Part model, mm, in its own coordinate system. Give positions to 0.01 mm unless a question says otherwise; leave off trailing zeros. Answer as a JSON object with one key per item and string values.
from build123d import *

# Parameters (mm, degrees)
SKETCH_1_R      = 2.5
SKETCH_1_W      = 3.3
SKETCH_1_H      = 3.3
EXTRUDE_1_DEPTH = 1445


with BuildPart() as part:
    # Эскиз1 → Бобышка-Вытянуть1 (new body)
    with BuildSketch(Plane.XY):
        Polygon((-10, 10), (-4.75, 10), (-3.1, 8), (-4.95, 8), (-4.95, 5.85), (-2.6, 3.5), (2.6, 3.5), (4.95, 5.85), (4.95, 8), (3.1, 8), (4.75, 10), (10, 10), (10, 4.75), (8, 3.1), (8, 4.95), (5.85, 4.95), (3.5, 2.6), (3.5, -2.6), (5.85, -4.95), (8, -4.95), (8, -3.1), (10, -4.75), (10, -10), (4.75, -10), (3.1, -8), (4.95, -8), (4.95, -5.85), (2.6, -3.5), (-2.6, -3.5), (-4.95, -5.85), (-4.95, -8), (-3.1, -8), (-4.75, -10), (-10, -10), (-10, -4.75), (-8, -3.1), (-8, -4.95), (-5.85, -4.95), (-3.5, -2.6), (-3.5, 2.6), (-5.85, 4.95), (-8, 4.95), (-8, 3.1), (-10, 4.75), align=None)
        Circle(SKETCH_1_R, mode=Mode.SUBTRACT)
        with Locations((-7.5, 7.5)):
            Rectangle(SKETCH_1_W, SKETCH_1_H, mode=Mode.SUBTRACT)
        with Locations((7.5, 7.5)):
            Rectangle(SKETCH_1_W, SKETCH_1_H, mode=Mode.SUBTRACT)
        with Locations((7.5, -7.5)):
            Rectangle(SKETCH_1_W, SKETCH_1_H, mode=Mode.SUBTRACT)
        with Locations((-7.5, -7.5)):
            Rectangle(SKETCH_1_W, SKETCH_1_H, mode=Mode.SUBTRACT)
    extrude(amount=-EXTRUDE_1_DEPTH)


solid = part.part
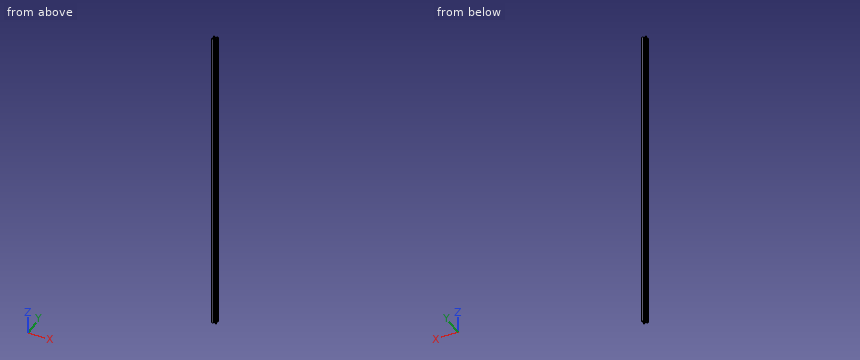
1. Cut at A-A on z = -617.5. State how many separate pieces and enclosed holes the cut face has, plus the area to 3 significant figures.
Worked answers:
{"separate pieces": "1", "enclosed holes": "5", "area": "118 mm^2"}
2. Pin check, flat tips, straight feed: P1, Ø3, axis at x = -2.5, z = -476, coming from the -Y side; P2, Ø1.6, axis at y = 1, z = -789.5, coming from the +X side; P3, Ø4, axis at y = 0.5, z = -952, coming from the -X side. Stop position of each tip, or through.
Worked answers:
{"P1": "stops at y = -9.09", "P2": "stops at x = 3.5", "P3": "stops at x = -3.5"}
3. Probe line 1 along X through (y, z) = (-4.25, -409); line 2 along X through (y, z) = (-7.25, -761). List the from-to ranges inside material, lowest first.
Worked answers:
{"line 1": "x = -9.39 to -8, -5.15 to -3.35, 3.35 to 5.15, 8 to 9.39", "line 2": "x = -10 to -9.15, -5.85 to -4.95, 4.95 to 5.85, 9.15 to 10"}
